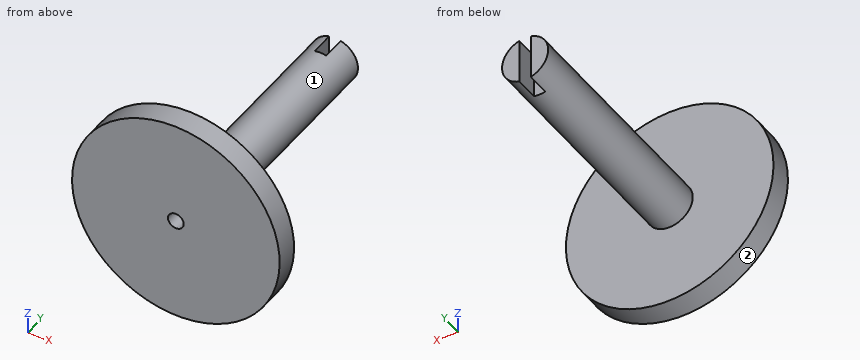
from build123d import *

# Parameters (mm, degrees)
SKETCH2_R                        = 57.15
BOSS_EXTRUDE1_DEPTH              = 12.7
SKETCH3_R                        = 12.7
BOSS_EXTRUDE2_DEPTH              = 127
CUT_EXTRUDE1_DEPTH               = 162.394965845
CUT_EXTRUDE1_DEPTH_BACK          = 162.394965845
SKETCH4_W                        = 6.35
SKETCH4_H                        = 12.7
F_5_8_0_341_DIAMETER_HOLE1_D     = 8.6614
F_5_8_0_341_DIAMETER_HOLE1_DEPTH = 22.797852917
F_5_8_0_341_DIAMETER_HOLE1_TIP   = 2.602147083


with BuildPart() as part:
    # Sketch2 → Boss-Extrude1 (new body)
    with BuildSketch(Plane(origin=(0, 0, 0), x_dir=(1, 0, 0), z_dir=(0, 1, 0))):
        with Locations(Location((0, 0, 0), (0, 0, 270))):
            Circle(SKETCH2_R)
    extrude(amount=BOSS_EXTRUDE1_DEPTH)

    # Sketch3 → Boss-Extrude2 (add)
    with BuildSketch(Plane(origin=(0, 12.7, 0), x_dir=(1, 0, 0), z_dir=(0, 1, 0))):
        with Locations(Location((0, 0, 0), (0, 0, 270))):
            Circle(SKETCH3_R)
    extrude(amount=BOSS_EXTRUDE2_DEPTH)

    # Sketch4 → Cut-Extrude1 (cut, two sides: drawn at the far end of the back side and taken through both)
    with BuildSketch(Plane.XY.offset(-CUT_EXTRUDE1_DEPTH_BACK)):
        with Locations((0, 133.35)):
            Rectangle(SKETCH4_W, SKETCH4_H)
    extrude(amount=CUT_EXTRUDE1_DEPTH + CUT_EXTRUDE1_DEPTH_BACK, mode=Mode.SUBTRACT)

    # 5/8 (0.341) Diameter Hole1
    with Locations(Plane(origin=(0, 0, 0), x_dir=(-1, 0, 0), z_dir=(0, -1, 0))):
        with Locations((0, 0)):
            Hole(F_5_8_0_341_DIAMETER_HOLE1_D / 2, depth=F_5_8_0_341_DIAMETER_HOLE1_DEPTH)
            with Locations((0, 0, -(F_5_8_0_341_DIAMETER_HOLE1_DEPTH + F_5_8_0_341_DIAMETER_HOLE1_TIP / 2))):  # 118° drill point
                Cone(0, F_5_8_0_341_DIAMETER_HOLE1_D / 2, F_5_8_0_341_DIAMETER_HOLE1_TIP, mode=Mode.SUBTRACT)


solid = part.part
Could you check a few things on this model? Use its own coordinates, in mm. Face numbers are marked on the shaded views. A direction names the side the tool comes from. Give positions to 0.01 mm unless a question says otherwise; leave off trailing zeros. Write each loop counter-clockwise with the first axis right and the second up, starting at its lowest first coordinate (ties: lowest second). Pieces come first, ordered by that corner, then holes. Notation, with made-up numbers: (63, -27.75) -> (102, -27.75) arc R11 ccw to (102, -8.75) -> close; hole circle Ø4 at (89.25, 31). An arc over 180 degrees is marked (long way). Write each question's results on one line, items separated by ' | '. Start each with the question number.
Q1. I'm going to push flat-ended pins straight in: pin 1 Ø4 at (y, z) = (36.5, 5) entering from +X; pin 2 Ø3 at (x, y) = (9, 73.5) entering from +Z; pin 3 Ø4 at (y, z) = (136, 4.5) entering from -X. Where does each tip first touch, or does it pass through?
Q2. Suppose I cut it at C-C, the plane z = -39. List the corners of the cut face in (x, y) for me, and give its area (3 significant figures).
Q3. Which directions (+Z, -Z, +X, -X, +Y, -Y) give clear straight access to the entire face, cutting with the end or side of a thin tool? Please do the marked faces 1 and 2.
Q4. Suppose I cut it at A-A, the plane y = 108.5. List the corners of the cut face in (x, z) for me, and give its area (3 significant figures).
Q5. I need wall thicknesses on probe 1 along Y at (x, z) = (1.5, -7); probe 2 along Y at (x, z) = (17, -9); probe 3 along Z at (x, y) = (0, 15.25). Which ranges of each line are inside material? Lowest first, please.
Q6. Suppose I cut it at B-B, the plane x = -23. List the corners of the cut face in (y, z) for me, and give its area (3 significant figures).
Outcome:
1) pin 1: x = 12.34 | pin 2: z = 10.25 | pin 3: x = -12.45
2) outline: (-41.77, 0) -> (41.77, 0) -> (41.77, 12.7) -> (-41.77, 12.7) -> close | area: 1,060 mm2
3) face 1: +Y | face 2: +Y, -Y
4) outline: circle Ø25.4 at (0, 0) | area: 507 mm2
5) probe 1: 0 to 127 | probe 2: 0 to 12.7 | probe 3: -12.7 to -4.33, 4.33 to 12.7
6) outline: (0, -52.32) -> (12.7, -52.32) -> (12.7, 52.32) -> (0, 52.32) -> close | area: 1,330 mm2
